Work out the finished part from the listing and answer in its coordinate system (mm). A direction names the side the tool comes from. Round coordinates to 2 decimals unless told otherwise and drop trailing zeros. One line per question, with ' | ' between items. Start each with the question number.
```python
from build123d import *

# Parameters (mm, degrees)
F0_W     = 81
F0_H     = 6
F1_DEPTH = 3
F3_R     = 2.99999
F2_W     = 9
F2_H     = 9
F2_W_2   = 6
F2_H_2   = 6
F4_DEPTH = 3
F5_R     = 4.49999
F6_R     = 4
F7_DEPTH = 4
F8_R     = 1.5


# Not quite as in the source:
# - a fillet or chamfer is up to 0.001 mm smaller than in the source, because OpenCascade refuses the exact size
# - ends of sketch curves that miss each other by under 0.0002 mm in the source are joined


with BuildPart() as f1:
    # F0 (on Top) → F1 (new body, symmetric)
    with BuildSketch(Plane.XY):
        Rectangle(F0_W, F0_H)
    extrude(amount=F1_DEPTH, both=True)

    # F3 (radius 3 in the source; OpenCascade refuses exactly that, so slightly less here)
    f3_edges = [f1.edges().sort_by_distance(p)[0] for p in [
        (0, -3, 3),
        (0, -3, -3),
        (0, 3, 3),
        (0, 3, -3),
    ]]
    fillet(f3_edges, radius=F3_R)

    # F2 (on face) → F4 (join)
    with BuildSketch(Plane.YZ.offset(40.5)):
        Rectangle(F2_W, F2_H)
        Rectangle(F2_W_2, F2_H_2, mode=Mode.SUBTRACT)
        Rectangle(F2_W_2, F2_H_2)
    extrude(amount=F4_DEPTH)

    # F5 (radius 4.5 in the source; OpenCascade refuses exactly that, so slightly less here)
    f5_edges = [f1.edges().sort_by_distance(p)[0] for p in [
        (42, 4.5, 4.5),
        (42, -4.5, 4.5),
        (42, -4.5, -4.5),
        (42, 4.5, -4.5),
    ]]
    fillet(f5_edges, radius=F5_R)

    # F6 (on face) → F7 (join)
    with BuildSketch(Plane(origin=(-40.5, 0, 0), x_dir=(0, -1, 0), z_dir=(-1, 0, 0))):
        Circle(F6_R)
        with BuildLine():
            ThreePointArc((-1e-05, -3), (-2.1213232725, -2.1213232725), (-3, -1e-05))
            ThreePointArc((-3, -1e-05), (-2.1213232725, 2.1213232725), (-1e-05, 3))
            ThreePointArc((-1e-05, 3), (2.1213232725, 2.1213232725), (3, 1e-05))
            ThreePointArc((3, 1e-05), (2.1213232725, -2.1213232725), (-1e-05, -3))
        make_face(mode=Mode.SUBTRACT)
        with BuildLine():
            ThreePointArc((-1e-05, 3), (-2.1213232725, 2.1213232725), (-3, 1e-05))
            ThreePointArc((-3, 1e-05), (-2.1213232725, -2.1213232725), (-1e-05, -3))
            ThreePointArc((-1e-05, -3), (2.1213232725, -2.1213232725), (3, -1e-05))
            ThreePointArc((3, -1e-05), (2.1213232725, 2.1213232725), (-1e-05, 3))
        make_face()
    extrude(amount=F7_DEPTH)

    # F8
    f8_edges = [f1.edges().sort_by_distance(p)[0] for p in [
        (-44.5, 4, 0),
    ]]
    fillet(f8_edges, radius=F8_R)


solid = f1.part
```
(1) For faces 5 (the cylindrical face through (0.57, 2.1, 2.14)), 6 (the cylindrical face through (0.57, -2.1, -2.14)), 7 (the cylindrical face through (42.021, -3.217, -3.147)), 8 (the cylindrical face through (0.57, 2.14, -2.1)), 9 (the flat face through (40.5, 1, -3)), determine the directions among +Z, -Z, +X, -X, +Y, -Y from which every point of the face is accessible in a straight line to the end or side of a thin tool.
(2) Given pin 1 Ø1 at (x, z) = (30, 3) entering from +Y; pin 2 Ø4 at (x, z) = (-4.5, 1) entering from +Y; pin 3 Ø3 at (y, z) = (3, 3.5) entering from +X, each flat-ended and moving along its own axis, determine where each tip first touches the part or whether it passes through.
(3) The mould has two halves that part along X. Classify faces 1 (the cylindrical face through (0.57, -2.1, 2.14)), 2 (the flat face through (-40.5, -1, 3)), 3 (the flat face through (-44.5, 0, 0)), 4 (the cylindrical face through (-41.732, 0.867, -3.905)): +X half, -X half, draft (parallel to the pull), parting line (faces both ways), or undercut.
(4) Consider L1, parallel to Z at x = 4, y = -0.25; L2, parallel to X at y = 4.25, z = 0.5; L3, parallel to X at y = 1.5, z = 3. Determine where each line is inside the solid, lowest interval first.
Returned:
1) face 5: +Z, +Y | face 6: -Z, -Y | face 7: -Z, +X, -X, -Y | face 8: -Z, +Y | face 9: -Z, +Y
2) pin 1: y = 1.66 | pin 2: y = 3 | pin 3: x = 43.5
3) face 1: undercut | face 2: undercut | face 3: -X half | face 4: draft
4) L1: -2.99 to 2.99 | L2: 40.5 to 43.5 | L3: -44.23 to -40.5, 40.5 to 43.5
